from build123d import *

# Parameters (mm, degrees)
F1_DEPTH = 0.8
F4_DEPTH = 1
F6_R     = 1.1
F7_DEPTH = 0.801


with BuildPart() as f1:
    # F0 (on Top) → F1 (new body)
    with BuildSketch(Plane.XY):
        Polygon((-8.5, 2.5), (-8.5, -27.5), (8.5, -27.5), (8.5, 2.5), (22.5, 2.5), (22.5, 22.5), (-22.5, 22.5), (-22.5, 2.5), align=None)
    extrude(amount=F1_DEPTH)

    # F3 (on offset) → F4 (join)
    with BuildSketch(Plane.YZ.offset(8)):
        with BuildLine():
            Line((18.5, 3.1), (18.5, 0.8))
            Line((18.5, 0.8), (22.5, 0.8))
            Line((22.5, 0.8), (22.5, 3.1))
            ThreePointArc((22.5, 3.1), (20.5, 5.1), (18.5, 3.1))
        make_face()
    extrude(amount=F4_DEPTH)

    # F5: F1 across plane


with BuildPart() as f1_1:
    add(f1.part)
    add(f1.part.mirror(Plane.YZ))

    # F6 (on face) → F7 (cut, through all)
    with BuildSketch(Plane.XY.offset(0.8)):
        with Locations((0, 15.5)):
            Circle(F6_R)
        with Locations((0, 7.5)):
            Circle(F6_R)
        with Locations((0, -16.5)):
            Circle(F6_R)
        with Locations((0, -20.5)):
            Circle(F6_R)
    extrude(amount=-F7_DEPTH, mode=Mode.SUBTRACT)


solid = f1_1.part
Check sheet for the modelled part. Datum: model origin and axes. Units: mm. A direction names the side the tool comes from. Give positions to 0.01 mm unless a question says otherwise; leave off trailing zeros. Order: outer loops, then holes, each group sorted by start corner. A loop starts at its lowest first (then second) coordinate and runs counter-clockwise, first axis right, second up. Notation, with made-up numbers: M 41.5,53 L 97.5,53 A25 cw 97.5,72 Z; hole C 49.25,-39 d2. An arc over 180 degrees is marked long. Answer as CSV lines item,"result". Start each with the question number.
Item 1: Cross-section at B-B on x = 0. Enter the section's corners in (y, z), plus the area to 3 significant figures.
Item 2: Tool access check on faces 1 (the face through (8, 20, 3)), 2 (the face through (9, 20, 3)), 3 (the face through (-0.238, -21.574, 0.406)). Record the directions out of +Z, -Z, +X, -X, +Y, -Y that give a thin tool (end or side, any length) a straight path to the whole face; none if there is none.
Item 3: Cross-section at A-A on y = 7.5. Enter the section's corners in (x, z).
Item 4: Gauge pin test, flat ends, axial feed: P1, Ø1.5, axis at x = 2.5, y = -17.5, coming from the +Z side; P2, Ø1.2, axis at y = 21, z = 2.5, coming from the +X side; P3, Ø1.1, axis at x = 8.5, z = 2, coming from the -Y side. Record the tip position at first contact, or that the pin passes through.
Item 5: Cross-section at D-D on y = -20.5. Enter the section's corners in (x, z).
Item 6: Mould release check, pull along X, two halves, no side actions. Record for faces 4 (the face through (0, 3, 0)), 5 (the face through (-0.238, 14.426, 0.406)), 6 (the face through (-8, 20, 3)), 7 (the face through (-9, 20, 3)): +X half, -X half, draft (parallel to the pull), parting line (faces both ways), or undercut.
Item 7: Cross-section at C-C on y = 20.5. Enter the section's corners in (x, z).
Item 8: Thickness scan on line 1 (Y direction, x = 0, z = 0.6); line 2 (X direction, y = 20.5, z = 4.25); line 3 (Z direction, x = -1, y = 14.5). Record the ranges inside material, lowest first. Write a range as [from, to].
Established:
1,outline,"M -27.5,0 L -21.6,0 L -21.6,0.8 L -27.5,0.8 Z; M -19.4,0 L -17.6,0 L -17.6,0.8 L -19.4,0.8 Z; M -15.4,0 L 6.4,0 L 6.4,0.8 L -15.4,0.8 Z; M 8.6,0 L 14.4,0 L 14.4,0.8 L 8.6,0.8 Z; M 16.6,0 L 22.5,0 L 22.5,0.8 L 16.6,0.8 Z"
1,area,"33.0 mm^2"
2,face 1,"+Z, +Y, -Y"
2,face 2,"+Z, +X, +Y, -Y"
2,face 3,"+Z, -Z"
3,outline,"M -22.5,0 L -1.1,0 L -1.1,0.8 L -22.5,0.8 Z; M 1.1,0 L 22.5,0 L 22.5,0.8 L 1.1,0.8 Z"
4,P1,"stops at z = 0.8"
4,P2,"stops at x = 9"
4,P3,"stops at y = 18.5"
5,outline,"M -8.5,0 L -1.1,0 L -1.1,0.8 L -8.5,0.8 Z; M 1.1,0 L 8.5,0 L 8.5,0.8 L 1.1,0.8 Z"
6,face 4,"draft"
6,face 5,"undercut"
6,face 6,"undercut"
6,face 7,"-X half"
7,outline,"M -22.5,0 L 22.5,0 L 22.5,0.8 L 9,0.8 L 9,5.1 L 8,5.1 L 8,0.8 L -8,0.8 L -8,5.1 L -9,5.1 L -9,0.8 L -22.5,0.8 Z"
8,line 1,"y = [-27.5, -21.6], [-19.4, -17.6], [-15.4, 6.4], [8.6, 14.4], [16.6, 22.5]"
8,line 2,"x = [-9, -8], [8, 9]"
8,line 3,"z = [0, 0.8]"
